Autodesk Fusion 360 part; units mm, degrees
sketch "Sketch1" plane through (0, 0, 0) normal (0, 1, 0) x (1, 0, 0)
  line L0 (0, 0) -> (50, 0)
  line L1 (50, 3) -> (0, 3)
  line L2 (0, 3) -> (0, 0)
  line L3 (50, -13) -> (0, -13)
  line L4 (0, -16) -> (50, -16)
  line L5 (0, -23) -> (15, -23)
  line L6 (15, -23) -> (15, -26)
  line L7 (15, -26) -> (0, -26)
  arc A0 (0, -13) -> (0, -26) centre (0, -19.5) ccw
  arc A1 (0, -16) -> (0, -23) centre (0, -19.5) ccw
  arc A2 (50, -16) -> (50, 3) centre (50, -6.5) ccw
  arc A3 (50, -13) -> (50, 0) centre (50, -6.5) ccw
extrude "Extrude1" add sketch "Sketch1" along normal blind 10
fillet "Fillet1" radius 2 1 edges at (15, 0, 24.5)
fillet "Fillet2" radius 2 1 edges at (15, 10, 24.5)
fillet "Fillet3" radius 2 1 edges at (0, 0, -1.5)
fillet "Fillet4" radius 2 1 edges at (0, 10, -1.5)
Work out the finished part from the listing and answer in its coordinate system (mm). A direction names the side the tool comes from. Give positions to 0.01 mm unless a question says otherwise; leave off trailing zeros. Loops run counter-clockwise (first coordinate to the right, second up) from the corner with the lowest first, then second, coordinate; pieces in that order, holes last. Notation, with made-up numbers: (23, -4.5) -> (75, -4.5) arc R17 ccw to (75, 8.5) -> close; hole circle Ø10 at (55.5, 57). An arc over 180 degrees is marked (long way). Write item = value, one per line. Start each with the question number.
(1) Find section D-D on z = 24. Give the vertices of the cut face in (x, y), and give its area (3 significant figures).
(2) Find section A-A on x = 12. Give the vertices of the cut face in (y, z).
(3) Which of the six approach directions +Z, -Z, +X, -X, +Y, -Y give full straight-line access (tool end or side, diameter ignored) to faces 1 (the flat face through (25, 5, 0)), 2 (the flat face through (0, 5, -2)), 3 (the flat face through (25, 5, 16))?
(4) Find section B-B on y = 4.5. Give the vertices of the cut face in (x, z).
(5) Find the intervals of material crossed by probe 1 along Z at (x, y) = (6.5, 4.5); probe 2 along Z at (x, y) = (21.5, 8.25); probe 3 along X at (y, z) = (6.5, 19.5), in increasing order. Write a range as from..to.
(6) Find section C-C on x = 30.5. Give the vertices of the cut face in (y, z), and give its area (3 significant figures).
(7) Given pin 1 Ø1 at (y, z) = (4, 7.5) entering from -X; pin 2 Ø1.5 at (y, z) = (5.5, -2) entering from -X; pin 3 Ø5 at (x, y) = (17, 5.5) entering from +Z; pin 4 Ø6 at (y, z) = (5, 6) entering from -X, each flat-ended and moving along its own axis, determine where each tip first touches the part or whether it passes through.
(8) The mould has two halves that part along Z. Classify faces 4 (the cylindrical face through (-3.5, 4.9, 19.6)), 5 (the cylindrical face through (59.498, 4.93, 6.291)), 6 (the flat face through (15, 5, 24)), 7 (the cylindrical face through (56.5, 4.9, 6.4)): +Z half, -Z half, draft (parallel to the pull), parting line (faces both ways), or undercut.
From the geometry:
q1.outline = (-4.69, 0) -> (13, 0) arc R2 ccw to (15, 2) -> (15, 8) arc R2 ccw to (13, 10) -> (-4.69, 10) -> close
q1.area = 195 mm^2
q2.outline = (0, -3) -> (10, -3) -> (10, 0) -> (0, 0) -> close; (0, 13) -> (10, 13) -> (10, 16) -> (0, 16) -> close; (0, 23) -> (10, 23) -> (10, 26) -> (0, 26) -> close
q3.face_1 = -X, +Y, -Y
q3.face_2 = -Z, -X, +Y, -Y
q3.face_3 = +X, +Y, -Y
q4.outline = (0, -3) -> (50, -3) arc R9.5 ccw to (50, 16) -> (0, 16) arc R3.5 cw to (0, 23) -> (15, 23) -> (15, 26) -> (0, 26) arc R6.5 ccw to (0, 13) -> (50, 13) arc R6.5 cw to (50, 0) -> (0, 0) -> close
q5.probe_1 = -3..0, 13..16, 23..26
q5.probe_2 = -3..0, 13..16
q5.probe_3 = -6.5..-3.5
q6.outline = (0, -3) -> (10, -3) -> (10, 0) -> (0, 0) -> close; (0, 13) -> (10, 13) -> (10, 16) -> (0, 16) -> close
q6.area = 60.0 mm^2
q7.pin_1 = 56.32
q7.pin_2 = 0
q7.pin_3 = 26
q7.pin_4 = 55.48
q8.face_4 = undercut
q8.face_5 = parting line
q8.face_6 = draft
q8.face_7 = undercut
